```python
from build123d import *

# Parameters (mm, degrees)
SKETCH1_W               = 80
SKETCH1_H               = 60
BOSS_EXTRUDE1_DEPTH     = 30
FILLET1_R               = 10
SKETCH2_R               = 1.5
CUT_EXTRUDE1_DEPTH      = 59.309518948
CUT_EXTRUDE2_DEPTH      = 20
CUT_EXTRUDE3_DEPTH      = 59.309518948
CUT_EXTRUDE3_DEPTH_BACK = 59.309518948
SKETCH4_R               = 1.5
SKETCH7_W               = 19.255318266
SKETCH7_H               = 12.5
CUT_EXTRUDE5_DEPTH      = 59.309518948
FILLET2_R               = 10
CUT_EXTRUDE6_DEPTH      = 20
FILLET4_R               = 4
SKETCH9_W               = 6.759025402
SKETCH9_H               = 6.458754369
CUT_EXTRUDE7_DEPTH      = 85.866070959


with BuildPart() as part:
    # Sketch1 → Boss-Extrude1 (new body)
    with BuildSketch(Plane(origin=(0, 0, 0), x_dir=(1, 0, 0), z_dir=(0, 1, 0))):
        Rectangle(SKETCH1_W, SKETCH1_H)
    extrude(amount=BOSS_EXTRUDE1_DEPTH)

    # Fillet1
    fillet1_edges = [part.edges().sort_by_distance(p)[0] for p in [
        (40, 15, 30),
        (40, 15, -30),
    ]]
    fillet(fillet1_edges, radius=FILLET1_R)

    # Sketch2 → Cut-Extrude1 (cut, through all)
    with BuildSketch(Plane(origin=(0, 30, 0), x_dir=(1, 0, 0), z_dir=(0, 1, 0))):
        with Locations(Location((-3.5, 15.5, 0), (0, 0, 270))):
            Circle(SKETCH2_R)
        with Locations(Location((27.5, 15.5, 0), (0, 0, 270))):
            Circle(SKETCH2_R)
        with Locations(Location((-3.5, -15.5, 0), (0, 0, 270))):
            Circle(SKETCH2_R)
        with Locations(Location((27.5, -15.5, 0), (0, 0, 270))):
            Circle(SKETCH2_R)
    extrude(amount=-CUT_EXTRUDE1_DEPTH, mode=Mode.SUBTRACT)

    # Sketch3 → Cut-Extrude2 (cut)
    with BuildSketch(Plane(origin=(0, 30, 0), x_dir=(1, 0, 0), z_dir=(0, 1, 0))):
        Polygon((-9.5, 17.5), (-5.5, 21.5), (29.5, 21.5), (33.5, 17.5), (33.5, -17.5), (29.5, -21.5), (-5.5, -21.5), (-9.5, -17.5), align=None)
    extrude(amount=-CUT_EXTRUDE2_DEPTH, mode=Mode.SUBTRACT)

    # Sketch4 → Cut-Extrude3 (cut, two sides: drawn at the far end of the back side and taken through both)
    with BuildSketch(Plane(origin=(0, 30, 0), x_dir=(1, 0, 0), z_dir=(0, 1, 0)).offset(-CUT_EXTRUDE3_DEPTH_BACK)):
        with Locations(Location((-32.5, 8.5, 0), (0, 0, 270))):
            Circle(SKETCH4_R)
        with Locations(Location((-32.5, -8.5, 0), (0, 0, 270))):
            Circle(SKETCH4_R)
    extrude(amount=CUT_EXTRUDE3_DEPTH + CUT_EXTRUDE3_DEPTH_BACK, mode=Mode.SUBTRACT)

    # Sketch7 → Cut-Extrude5 (cut, through all)
    with BuildSketch(Plane(origin=(0, 30, 0), x_dir=(1, 0, 0), z_dir=(0, 1, 0))):
        with Locations((-30.372340867, 23.75)):
            Rectangle(SKETCH7_W, SKETCH7_H)
        with Locations((-30.372340867, -23.75)):
            Rectangle(SKETCH7_W, SKETCH7_H)
    extrude(amount=-CUT_EXTRUDE5_DEPTH, mode=Mode.SUBTRACT)

    # Fillet2
    fillet2_edges = [part.edges().sort_by_distance(p)[0] for p in [
        (-20.744681734, 15, 30),
        (-40, 15, 17.5),
        (-20.744681734, 15, -30),
        (-40, 15, -17.5),
    ]]
    fillet(fillet2_edges, radius=FILLET2_R)

    # Sketch8 → Cut-Extrude6 (cut)
    with BuildSketch(Plane.XZ):
        with BuildLine():
            Line((-17.426212782, 27.440238091), (-17.426212782, -27.440238091))
            ThreePointArc((-17.426212782, -27.440238091), (-19.877460897, -24.073370197), (-20.744681734, -20))
            Line((-20.744681734, -20), (-20.744681734, -17.5))
            Line((-20.744681734, -17.5), (-30, -17.5))
            ThreePointArc((-30, -17.5), (-37.071067812, -14.571067812), (-40, -7.5))
            Line((-40, -7.5), (-40, 7.5))
            ThreePointArc((-40, 7.5), (-37.071067812, 14.571067812), (-30, 17.5))
            Line((-30, 17.5), (-20.744681734, 17.5))
            Line((-20.744681734, 17.5), (-20.744681734, 20))
            ThreePointArc((-20.744681734, 20), (-19.877460897, 24.073370197), (-17.426212782, 27.440238091))
        make_face()
    extrude(amount=-CUT_EXTRUDE6_DEPTH, mode=Mode.SUBTRACT)

    # Fillet4
    fillet4_edges = [part.edges().sort_by_distance(p)[0] for p in [
        (-17.426212782, 10, 27.440238091),
        (-17.426212782, 10, -27.440238091),
    ]]
    fillet(fillet4_edges, radius=FILLET4_R)

    # Sketch9 → Cut-Extrude7 (cut, through all)
    with BuildSketch(Plane.ZY.offset(-33.5)):
        with Locations((0, 13.888622085)):
            Rectangle(SKETCH9_W, SKETCH9_H)
    extrude(amount=-CUT_EXTRUDE7_DEPTH, mode=Mode.SUBTRACT)


solid = part.part
```
Geometry: final body of the model. Coordinates: model frame, mm. A direction names the side the tool comes from. Round coordinates to 2 decimals unless told otherwise and drop trailing zeros. Order: outer loops, then holes, each group sorted by start corner. A loop starts at its lowest first (then second) coordinate and runs counter-clockwise, first axis right, second up. Notation, with made-up numbers: (11.5, -10.75) -> (65.5, -10.75) arc R4 ccw to (65.5, -6.75) -> close; hole circle Ø4 at (35, 22). An arc over 180 degrees is marked (long way). Write each question's results on one line, items separated by ' | '.
Q1. Section query C-C (z = -15.5). Output: boundary loops of the cut face in (x, y).
Response values:
outline: (-36, 20) -> (-17.43, 20) -> (-17.43, 0) -> (-5, 0) -> (-5, 10) -> (-9.5, 10) -> (-9.5, 30) -> (-36, 30) -> close; (-2, 0) -> (26, 0) -> (26, 10) -> (-2, 10) -> close; (29, 0) -> (40, 0) -> (40, 30) -> (33.5, 30) -> (33.5, 10) -> (29, 10) -> close
Q2. Section query D-D (x = 18.5). Output: boundary loops of the cut face in (y, z), and give its area (3 significant figures).
Response values:
outline: (0, -30) -> (30, -30) -> (30, -21.5) -> (10, -21.5) -> (10, 21.5) -> (30, 21.5) -> (30, 30) -> (0, 30) -> close | area: 940 mm²
Q3. Ray query, line 1 along X through (y, z) = (3, -15.5); line 2 along Z through (x, y) = (8, 22.75); line 3 along X through (y, z) = (19.5, 5). Return the intervals inside material, ascending.
Response values:
line 1: -17.43 to -5, -2 to 26, 29 to 40 | line 2: -30 to -21.5, 21.5 to 30 | line 3: -17.43 to -9.5, 33.5 to 40
Q4. Section query B-B (y = 24.25). Output: boundary loops of the cut face in (x, z), and give its area (3 significant figures).
Response values:
outline: (-40, -7.5) arc R10 ccw to (-30, -17.5) -> (-20.74, -17.5) -> (-20.74, -20) arc R10 ccw to (-10.74, -30) -> (30, -30) arc R10 ccw to (40, -20) -> (40, 20) arc R10 ccw to (30, 30) -> (-10.74, 30) arc R10 ccw to (-20.74, 20) -> (-20.74, 17.5) -> (-30, 17.5) arc R10 ccw to (-40, 7.5) -> close; hole circle Ø3 at (-32.5, -8.5); hole circle Ø3 at (-32.5, 8.5); hole (-9.5, -17.5) -> (-5.5, -21.5) -> (29.5, -21.5) -> (33.5, -17.5) -> (33.5, 17.5) -> (29.5, 21.5) -> (-5.5, 21.5) -> (-9.5, 17.5) -> close | area: 2,360 mm²
Q5. Pull-direction query (Y, two-part tool) for faces 1 (the face through (-18, 30, 0)), 2 (the face through (-17.426, 10, 0)), 3 (the face through (11, 0, 0)), 4 (the face through (37, 17.118, 0)); classes: released by +Y, released by -Y, zero draft, split by the parting line, or undercut.
Response values:
face 1: released by +Y | face 2: zero draft | face 3: released by -Y | face 4: undercut
Q6. Access query for faces 5 (the face through (-20.745, 25, 19)), 6 (the face through (-16.81, 10.14, 27.5)), 7 (the face through (37, 14, 3.38)), 8 (the face through (-16.845, 10.14, -27.444)). Directions: +Z, -Z, +X, -X, +Y, -Y. A direction counts if a zero-diameter tool reaches every point of the face in a straight line with its end or side. Return the directions, or none.
Response values:
face 5: +Z, -X, +Y, -Y | face 6: +Z, -X, -Y | face 7: +X | face 8: -Z, -X, -Y
Q7. Section query A-A (z = 1.5). Output: boundary loops of the cut face in (x, y).
Response values:
outline: (-40, 20) -> (-17.43, 20) -> (-17.43, 0) -> (40, 0) -> (40, 10.66) -> (33.5, 10.66) -> (33.5, 10) -> (-9.5, 10) -> (-9.5, 30) -> (-40, 30) -> close; (33.5, 17.12) -> (40, 17.12) -> (40, 30) -> (33.5, 30) -> close
Q8. Pin query (flat end, axial travel): pin 1 Ø2.5 at (x, z) = (-32.5, 8.5) entering from -Y (3 decimals); pin 2 Ø2 at (y, z) = (17.5, -3.5) entering from -X; pin 3 Ø1.9 at (x, y) = (36.5, 14) entering from -Z; pin 4 Ø3 at (x, y) = (-26, 26) entering from -Z. Return the tip coordinate at first contact, or that it passes through.
Response values:
pin 1: through | pin 2: x = -17.43 | pin 3: z = -28.32 | pin 4: z = -17.5
